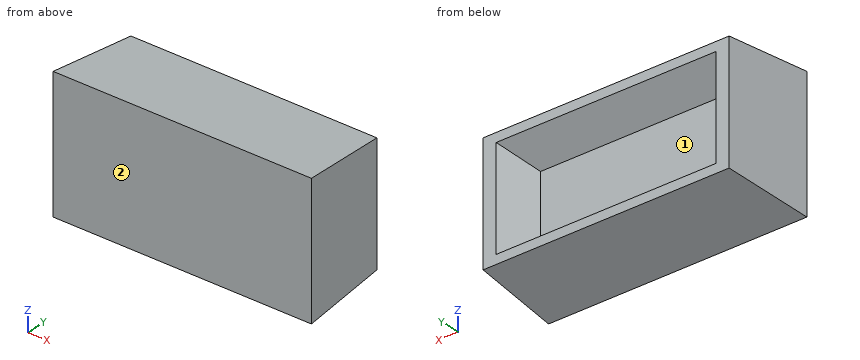
from build123d import *

# Parameters (mm, degrees)
SKETCH1_W           = 205.785682804
SKETCH1_H           = 104.534748446
BOSS_EXTRUDE1_DEPTH = 70.104
BOSS_EXTRUDE1_TAPER = 4
SKETCH2_W           = 145.758865666
SKETCH2_H           = 50.974097726
CUT_EXTRUDE1_DEPTH  = 25.4
DRAFT1_ANGLE        = 30


with BuildPart() as part:
    # Sketch1 → Boss-Extrude1 (new body)
    with BuildSketch(Plane(origin=(0, 0, 0), x_dir=(1, 0, 0), z_dir=(0, 1, 0))):
        Rectangle(SKETCH1_W, SKETCH1_H)
    extrude(amount=BOSS_EXTRUDE1_DEPTH, taper=BOSS_EXTRUDE1_TAPER)

    # Sketch2 → Cut-Extrude1 (cut)
    with BuildSketch(Plane(origin=(0, 70.104, 0), x_dir=(1, 0, 0), z_dir=(0, 1, 0))):
        Rectangle(SKETCH2_W, SKETCH2_H)
    extrude(amount=-CUT_EXTRUDE1_DEPTH, mode=Mode.SUBTRACT)

    # Draft1
    draft1_faces = [part.faces().sort_by_distance(p)[0] for p in [
        (0, 57.404, 25.487048863),
        (72.879432833, 57.404, 0),
        (0, 57.404, -25.487048863),
        (-72.879432833, 57.404, 0),
    ]]
    draft(draft1_faces, Plane.ZX.offset(44.704), DRAFT1_ANGLE)


solid = part.part
Can you work these out from the model? Positions are in its coordinate system, mm. Face numbers are marked on the shaded views. Coordinates: 2 decimals unless noted, no trailing zeros.
Q1. Please list where these lines run through material, in increasing order: L1, parallel to Y at x = 49, z = -18; L2, parallel to X at y = 55.5, z = -15.5; L3, parallel to Z at x = 30, y = 61.5.
Results found:
L1: y = 0 to 44.7
L2: x = -99.01 to -79.11, 79.11 to 99.01
L3: z = -47.97 to -35.18, 35.18 to 47.97
Q2. For P1, Ø1, axis at x = 3, y = 61.5, coming from the +Z side; P2, Ø8, axis at x = 20, z = 29, coming from the +Y side; P3, Ø12, axis at x = 29.5, z = 33, coming from the +Y side, each with a flat end and sliding along its axis, tell me the tip position at first contact or that it passes through.
Results found:
P1: stops at z = 48
P2: stops at y = 57.72
P3: stops at y = 68.11
Q3. If we mould it in two halves opening along Z, with no side actions, what happens to the marked faces 1 and 2? For each: +Z half, -Z half, draft (parallel to the pull), parting line (faces both ways), or undercut.
Results found:
face 1: undercut
face 2: draft
